Source: three-view drawing plus pictorial views. Frame: mm from the lowest corner of the part. A direction names the side the tool comes from. Coordinates: 2 decimals unless noted, no trailing zeros. Write each loop counter-clockwise with the first axis right and the second up, starting at its lowest first coordinate (ties: lowest second). Pieces come first, ordered by that corner, then holes. Notation, with made-up numbers: (10, 74.25) - (16, 74.25) arc R28 ccw to (16, 92.25) - close; hole circle Ø9 at (70.5, 19). An arc over 180 degrees is marked (long way). Answer as a JSON object with one key per item and string values. Group by question number.
Item 1: Set-up query: the marked faces 4 and 5. Return all of +Z, -Z, +X, -X, +Y, -Y with unobstructed straight access to the full face (end or side cutting, diameter ignored); none if empty.
Item 2: Section B-B on z = 8.25. Return loops of the section in (x, y), and give its area (3 significant figures).
Item 3: Section A-A on y = 22. Return loops of the section in (x, z).
Item 4: Section D-D on z = 22.75. Return loops of the section in (x, y).
Item 5: Mould query, pull axis Y, two halves, no side actions, for the marked faces 1, 2 and 3. Classes: pulls with the +Y half, pulls with the -Y half, needs draft (parallel to the pull), parting line crosses it, or undercut.
Item 6: First-contact query: pin 1 Ø8 at (x, z) = (22.5, 21.5) entering from +Y; pin 2 Ø10 at (x, z) = (33.5, 22.5) entering from +Y; pin 3 Ø2 at (x, z) = (6, 5.5) entering from -Y. Flat tips, straight axial feed; report the tip coordinate or a pass-through.
Item 7: Line query: line 1 along Y through (x, z) = (22, 8); line 2 along X through (y, z) = (21.5, 2.75); line 3 along Z through (x, y) = (33.5, 17). Output: solid intervals per line, ascending. Write a range as from..to.
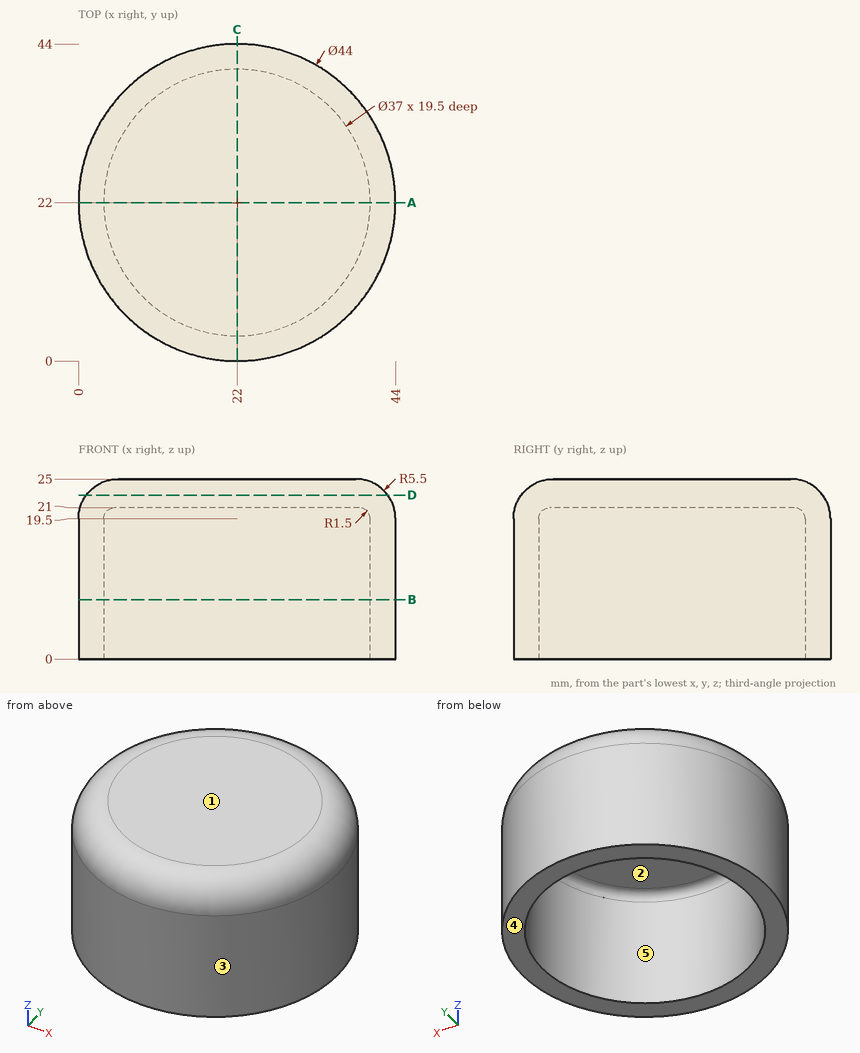
Checks:
{
 "1": {"face 4": "-Z, +X, -X, +Y, -Y", "face 5": "-Z"},
 "2": {"outline": "circle Ø44 at (22, 22); hole circle Ø37 at (22, 22)", "area": "445 mm^2"},
 "3": {"outline": "(0, 0) - (3.5, 0) - (3.5, 19.5) arc R1.5 cw to (5, 21) - (39, 21) arc R1.5 cw to (40.5, 19.5) - (40.5, 0) - (44, 0) - (44, 19.5) arc R5.5 ccw to (38.5, 25) - (5.5, 25) arc R5.5 ccw to (0, 19.5) - close"},
 "4": {"outline": "circle Ø41.87 at (22, 22)"},
 "5": {"face 1": "needs draft", "face 2": "undercut", "face 3": "parting line crosses it"},
 "6": {"pin 1": "y = 44", "pin 2": "y = 42.79", "pin 3": "y = 5.91"},
 "7": {"line 1": "0..3.5, 40.5..44", "line 2": "0.01..3.51, 40.49..43.99", "line 3": "21..25"}
}
